Drawing for the job (mm, zero at the part's lowest x, y, z). A direction names the side the tool comes from. Coordinates: 2 decimals unless noted, no trailing zeros. Write each loop counter-clockwise with the first axis right and the second up, starting at its lowest first coordinate (ties: lowest second). Pieces come first, ordered by that corner, then holes. Notation, with made-up numbers: (8, 12.5) -> (58, 12.5) arc R31 cw to (58, 41.5) -> close; hole circle Ø4 at (-29.75, 2.5). An arc over 180 degrees is marked (long way). Write each question's results on one line, items separated by ' | '. Start each with the question number.
Q1. Drill centre lines: line 1 (X direction, y = 0.6, z = 5); line 2 (Z direction, x = 38, y = 7.5). Where is each one in solid material? Low to high.
Q2. Two-plate mould, pull along Z, no slides. Class the marked faces 1, 2 and 3: released by +Z, released by -Z, zero draft, split by the parting line, or undercut.
Q3. Tool access for the marked faces 4 and 5: list every direction of +Z, -Z, +X, -X, +Y, -Y with a clear straight run to the whole face (end or side of a thin tool).
Q4. Saw through at A-A on y = 5. Give the cut face in (x, z), and give its area (3 significant figures).
Q5. Saw through at B-B on z = 3. Give the cut face in (x, y), and give its area (3 significant figures).
Q6. Saw through at C-C on x = 29. Give the cut face in (y, z).
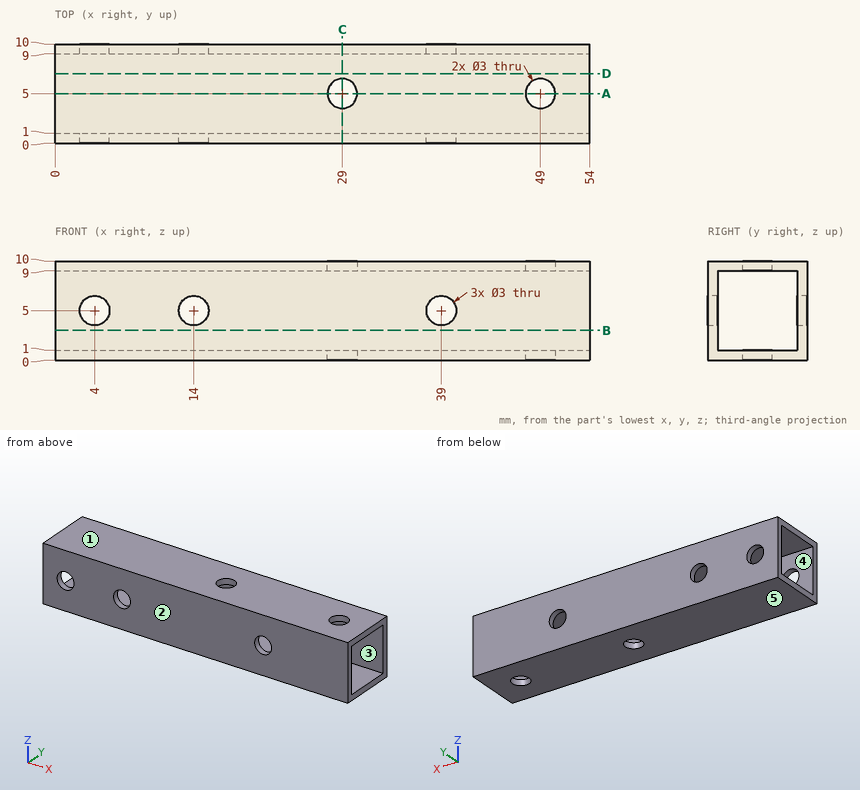
Returned:
1) line 1: x = 0 to 2.5, 5.5 to 12.5, 15.5 to 37.5, 40.5 to 54 | line 2: z = 0 to 1, 9 to 10
2) face 1: released by +Z | face 2: zero draft | face 3: undercut
3) face 4: +X, -X | face 5: -Z, +X, -X, +Y, -Y
4) outline: (0, 0) -> (27.5, 0) -> (27.5, 1) -> (0, 1) -> close; (0, 9) -> (27.5, 9) -> (27.5, 10) -> (0, 10) -> close; (30.5, 0) -> (47.5, 0) -> (47.5, 1) -> (30.5, 1) -> close; (30.5, 9) -> (47.5, 9) -> (47.5, 10) -> (30.5, 10) -> close; (50.5, 0) -> (54, 0) -> (54, 1) -> (50.5, 1) -> close; (50.5, 9) -> (54, 9) -> (54, 10) -> (50.5, 10) -> close | area: 96.0 mm2
5) outline: (0, 0) -> (54, 0) -> (54, 1) -> (0, 1) -> close; (0, 9) -> (54, 9) -> (54, 10) -> (0, 10) -> close | area: 108 mm2
6) outline: (0, 0) -> (3.5, 0) -> (3.5, 1) -> (1, 1) -> (1, 9) -> (3.5, 9) -> (3.5, 10) -> (0, 10) -> close; (6.5, 0) -> (10, 0) -> (10, 10) -> (6.5, 10) -> (6.5, 9) -> (9, 9) -> (9, 1) -> (6.5, 1) -> close
